Solid Edge part; units mm, degrees
sketch "Sketch1" plane through (-70.6437, 101.6, 0) normal (0, -1, 0) x (1, 0, 0)
  line L0 (-61.1187, -43.6562) -> (-46.8312, -43.6562)
  line L1 (-46.8312, -43.6562) -> (-46.8312, -24.6062)
  line L2 (-46.8312, -24.6062) -> (-61.1187, -24.6062)
  line L3 (-61.1187, -24.6062) -> (-61.1187, -43.6562)
  dimension "D1" = 46.8312
  dimension "D2" = 61.1187
extrude "Protrusion1" add sketch "Sketch1" along normal up to vertex (203.2 mm away)
sketch "Sketch2" plane through (-131.7625, 0, -34.1313) normal (-1, 0, 0) x (0, -1, 0)
  line L0 (-114.3, 9.525) -> (114.3, 9.525)
  line L1 (114.3, 9.525) -> (114.3, -9.525)
  line L2 (114.3, -9.525) -> (-114.3, -9.525)
  line L3 (-114.3, -9.525) -> (-114.3, 9.525)
extrude "Protrusion2" add sketch "Sketch2" along normal blind 4.7625
The listing builds one solid part. Answer for the finished solid, in the listing's coordinates (mm). A direction names the side the tool comes from. Coordinates: 2 decimals unless noted, no trailing zeros. Loops run counter-clockwise (first coordinate to the right, second up) from the corner with the lowest first, then second, coordinate; pieces in that order, holes last. Notation, with made-up numbers: M 20,-10 L 57,-10 A34 cw 57,22 Z; hole C 64.5,44.25 d1. An arc over 180 degrees is marked long. Answer as CSV lines item,"result". Start each with the question number.
(1) For faces 1 (the flat face through (-131.762, 108, -34)), 2 (the flat face through (-125, -101.6, -34)), 3 (the flat face through (-134, 114.3, -34)), determine the directions among +Z, -Z, +X, -X, +Y, -Y from which every point of the face is accessible in a straight line to the end or side of a thin tool.
(2) Given pin 1 (6.5 mm diameter, centred on y = 110, z = -37, fed in from +X); pin 2 (8 mm diameter, centred on x = -123, z = -28.5, fed in from +Y); pin 3 (4 mm diameter, centred on x = -131, z = -41.5, fed in from +Y), each flat-ended and moving along its own axis, determine where each tip first touches the part or whether it passes through.
(3) Find the intervals of material crossed by L1, parallel to Y at x = -122.75, z = -38.25, in increasing order. Write a range as [from, to].
(4) The part is cut by section B-B (x = -121.75). Give the vertices of the cut face in (y, z), and give its area (3 significant figures).
(5) The part is cut by section A-A (z = -41.25). Give the vertices of the cut face in (x, y) (1 decimal).
Determined:
1,face 1,"+Z, -Z, +X, +Y"
1,face 2,"+Z, -Z, +X, -Y"
1,face 3,"+Z, -Z, +X, -X, +Y"
2,pin 1,"x = -131.76"
2,pin 2,"y = 101.6"
2,pin 3,"y = 114.3"
3,L1,"[-101.6, 101.6]"
4,outline,"M -101.6,-43.66 L 101.6,-43.66 L 101.6,-24.61 L -101.6,-24.61 Z"
4,area,"3,870 mm2"
5,outline,"M -136.5,-114.3 L -131.8,-114.3 L -131.8,-101.6 L -117.5,-101.6 L -117.5,101.6 L -131.8,101.6 L -131.8,114.3 L -136.5,114.3 Z"
